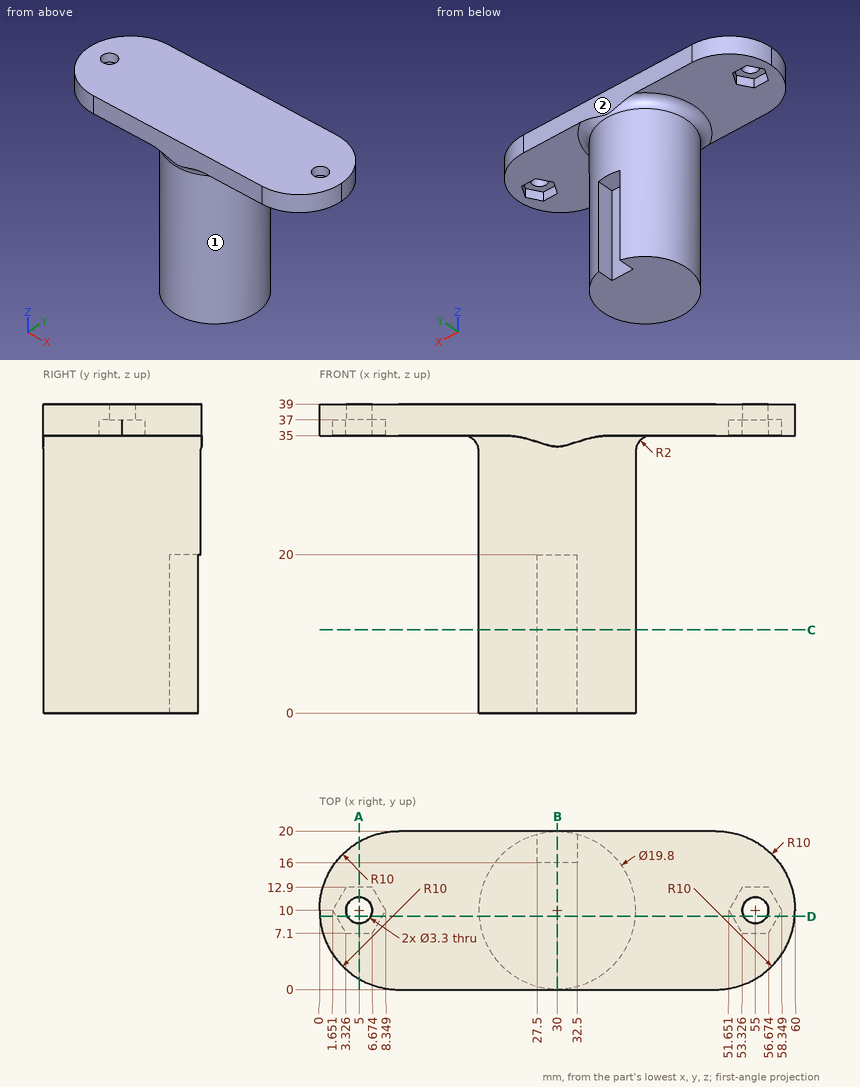
Design review of the part shown in the three views and the two pictorial views. Dimensions are in mm from the part's minimum x, y and z. A direction names the side the tool comes from. Give positions to 0.01 mm unless a question says otherwise; leave off trailing zeros. Loops run counter-clockwise (first coordinate to the right, second up) from the corner with the lowest first, then second, coordinate; pieces in that order, holes last. Notation, with made-up numbers: M 48,63 L 80,63 A28 ccw 80,81 Z; hole C 26.5,14 d9. An arc over 180 degrees is marked long. Answer as a JSON object with one key per item and string values.
Item 1: We need section A-A (x = 5). State the section outline as (y, z) points.
Output values:
{"outline": "M 1.34,35 L 7.1,35 L 7.1,37 L 8.35,37 L 8.35,39 L 1.34,39 Z; M 11.65,37 L 12.9,37 L 12.9,35 L 18.66,35 L 18.66,39 L 11.65,39 Z"}
Item 2: Machinability: for the marked faces 1 and 2, which of the approach directions +Z, -Z, +X, -X, +Y, -Y give a long, thin tool a straight path to every point of the face, cutting with its end or side? Answer none if there is none.
Output values:
{"face 1": "-Z", "face 2": "+Z, -Z, +X, -X, +Y"}
Item 3: We need section C-C (z = 10.5). State the section outline as (x, y) points, and give its area (3 significant figures).
Output values:
{"outline": "M 27.5,16 L 27.5,19.58 A9.9 ccw long 32.5,19.58 L 32.5,16 Z", "area": "289 mm2"}
Item 4: Wall thickness on line 1 along Z through (x, y) = (10, 14); line 2 along Y through (x, z) = (55, 38.5); line 3 along Z through (x, y) = (56, 12.25): over which ranges is each line inside the solid? List them lowest first.
Output values:
{"line 1": "z = 35 to 39", "line 2": "y = 1.34 to 8.35, 11.65 to 18.66", "line 3": "z = 37 to 39"}
Item 5: We need section D-D (y = 9.25). Count the separate pieces of the cut face and the enclosed holes in it.
Output values:
{"separate pieces": "3", "enclosed holes": "0"}
Item 6: For P1, Ø4, axis at x = 30, z = 7, coming from the +Y side; P2, Ø3, axis at x = 29, z = 26, coming from the -Y side; P3, Ø10, axis at x = 17, z = 19.5, coming from the -Y side, all flat-tipped, find the tip position at first contact; note any pin that passes through.
Output values:
{"P1": "stops at y = 16", "P2": "stops at y = 0.1", "P3": "stops at y = 4.17"}
Item 7: We need section B-B (x = 30). State the section outline as (y, z) points (1 decimal).
Output values:
{"outline": "M 0,33.6 A2 cw 0.1,33 L 0.1,0 L 16,0 L 16,20 L 19.9,20 L 19.9,33 A2 cw 20,33.6 L 20,39 L 0,39 Z"}
